The listing builds one solid part. Answer for the finished solid, in the listing's coordinates (mm). A direction names the side the tool comes from. Round coordinates to 2 decimals unless told otherwise and drop trailing zeros. Write each loop counter-clockwise with the first axis right and the second up, starting at its lowest first coordinate (ties: lowest second). Pieces come first, ordered by that corner, then holes. Notation, with made-up numbers: (77.25, 53.5) - (122.25, 53.5) arc R31 cw to (122.25, 82.5) - close; hole circle Ø3 at (-18.5, 82.25). An arc over 180 degrees is marked (long way). Answer in a Markdown table with one row per item.
from build123d import *

# Parameters (mm, degrees)
F1_DEPTH = 63.5
F2_DEPTH = 25.4
F3_DEPTH = 7.9375
F0_W     = 25.4
F0_H     = 19.05
F4_DEPTH = 25.4
F6_R     = 5.08


with BuildPart() as f1:
    # F0 (on Right) → F1 (new body, symmetric)
    with BuildSketch(Plane.YZ):
        Polygon((22.225, 9.525), (-41.275, 9.525), (-41.275, -9.525), (41.275, -9.525), (41.275, 9.525), align=None)
    extrude(amount=F1_DEPTH, both=True)

    # F0 (on Right) → F2 (join, symmetric)
    with BuildSketch(Plane.YZ):
        with BuildLine():
            Line((22.225, 27.0002), (22.225, 9.525))
            Line((22.225, 9.525), (41.275, 9.525))
            Line((41.275, 9.525), (41.275, 27.0002))
            ThreePointArc((41.275, 27.0002), (45.9246798487, 38.2255201513), (57.15, 42.8752))
            Line((57.15, 42.8752), (61.7728, 42.8752))
            Line((61.7728, 42.8752), (61.7728, 61.9252))
            Line((61.7728, 61.9252), (57.15, 61.9252))
            add(Edge.make_bspline(
                [(56.4704910637, 61.9185890322), (56.6978208401, 61.9216781998), (56.9243298896, 61.9238834244), (57.15, 61.9252)],
                knots=[110.8312649527, 110.8312649527, 110.8312649527, 110.8312649527, 111.5045361635, 111.5045361635, 111.5045361635, 111.5045361635], degree=3))
            ThreePointArc((56.4704910637, 61.9185890322), (32.2152103017, 51.4544815822), (22.225, 27.0002))
        make_face()
    extrude(amount=F2_DEPTH, both=True)

    # F0 (on Right) → F3 (join, symmetric)
    with BuildSketch(Plane.YZ):
        with BuildLine():
            add(Edge.make_bspline(
                [(-41.275, 9.525), (-40.6142083443, 36.9480472053), (19.0483552666, 61.4100623809), (56.4704910637, 61.9185890322)],
                knots=[0, 0, 0, 0, 110.8312649527, 110.8312649527, 110.8312649527, 110.8312649527], degree=3))
            Line((-41.275, 9.525), (22.225, 9.525))
            Line((22.225, 9.525), (22.225, 27.0002))
            ThreePointArc((22.225, 27.0002), (32.2152103017, 51.4544815822), (56.4704910637, 61.9185890322))
        make_face()
    extrude(amount=F3_DEPTH, both=True)

    # F0 (on Right) → F4 (join, symmetric)
    with BuildSketch(Plane.YZ):
        with Locations((74.4728, 52.4002)):
            Rectangle(F0_W, F0_H)
    extrude(amount=F4_DEPTH, both=True)

    # F0 (on Right) → F5 (revolve)
    with BuildSketch(Plane.YZ):
        Polygon((87.1728, 66.675), (87.1728, 61.9252), (87.1728, 42.8752), (87.1728, 38.1), (112.5728, 38.1), (112.5728, 66.675), align=None)
    revolve(axis=Axis((0, 87.1728, 52.3875), (0, 0, -1)))

    # F6
    f6_edges = [f1.edges().sort_by_distance(p)[0] for p in [
        (63.5, -41.275, 0),
        (63.5, 41.275, 0),
        (-63.5, 41.275, 0),
        (-63.5, -41.275, 0),
    ]]
    fillet(f6_edges, radius=F6_R)


solid = f1.part
(1) Find the intervals of material crossed by line 1 (X direction, y = -18.5, z = 22.5); line 2 (Z direction, x = 4.5, y = 69) (3 decimals); line 3 (Z direction, x = 32, y = -24) (3 decimals), in increasing order.
Checked values:
| item | result |
|---|---|
| line 1 | x = -7.94 to 7.94 |
| line 2 | z = 38.1 to 66.675 |
| line 3 | z = -9.525 to 9.525 |
(2) Flat-ended cylindrical pins translate along their axes: pin 1 (10 mm diameter, centred on x = 23, z = 33, fed in from +Y); pin 2 (19 mm diameter, centred on x = -15, z = 22, fed in from -Y); pin 3 (6 mm diameter, centred on x = -3.5, z = 39, fed in from +Y). Find the tip coordinate at first contact, or state that the pin passes through.
Checked values:
| item | result |
|---|---|
| pin 1 | stops at y = 45.7 |
| pin 2 | stops at y = -40.16 |
| pin 3 | stops at y = 112.57 |
(3) Section B-B (x = -32) is taken. Give the vertices of the cut face in (y, z) (3 decimals).
Checked values:
| item | result |
|---|---|
| outline | (-41.275, -9.525) - (41.275, -9.525) - (41.275, 9.525) - (-41.275, 9.525) - close |
(4) For faces 1 (the flat face through (25.4, 47, 42)), 2 (the flat face through (-25.4, 47, 42)), 3 (the flat face through (17, 22.225, 18)), 4 (the flat face through (-17, 22.225, 18)), determine the directions among +Z, -Z, +X, -X, +Y, -Y from which every point of the face is accessible in a straight line to the end or side of a thin tool.
Checked values:
| item | result |
|---|---|
| face 1 | +Z, +X, +Y, -Y |
| face 2 | +Z, -X, +Y, -Y |
| face 3 | +Z, +X, -Y |
| face 4 | +Z, -X, -Y |
(5) Section A-A (y = 76.5) is taken. Give the vertices of the cut face in (x, z) (3 decimals), and give its area (3 significant figures).
Checked values:
| item | result |
|---|---|
| outline | (-25.4, 42.875) - (-23.049, 42.875) - (-23.049, 38.1) - (23.049, 38.1) - (23.049, 42.875) - (25.4, 42.875) - (25.4, 61.925) - (23.049, 61.925) - (23.049, 66.675) - (-23.049, 66.675) - (-23.049, 61.925) - (-25.4, 61.925) - close |
| area | 1,410 mm2 |
